For this review, take the finished solid that the model builds, in its own axes (mm). Face numbers are marked on the shaded views. A direction names the side the tool comes from. Coordinates: 2 decimals unless noted, no trailing zeros. Write each loop counter-clockwise with the first axis right and the second up, starting at its lowest first coordinate (ties: lowest second). Pieces come first, ordered by that corner, then holes. Notation, with made-up numbers: M 54.5,74 L 80.5,74 A13 ccw 80.5,92 Z; hole C 80.5,-17 d10. An arc over 180 degrees is marked long. Return JSON: item names as keys, results as strings.
```python
from build123d import *

# Parameters (mm, degrees)
SKETCH1_W           = 40
SKETCH1_H           = 40
BOSS_EXTRUDE1_DEPTH = 40
CUT_EXTRUDE1_DEPTH  = 40
CUT_EXTRUDE2_DEPTH  = 40
CUT_EXTRUDE10_DEPTH = 40
CUT_EXTRUDE11_DEPTH = 40
CUT_EXTRUDE12_DEPTH = 40


with BuildPart() as part:
    # Sketch1 → Boss-Extrude1 (new body)
    with BuildSketch(Plane.XY):
        with Locations((20, 20)):
            Rectangle(SKETCH1_W, SKETCH1_H)
    extrude(amount=BOSS_EXTRUDE1_DEPTH)

    # Sketch2 → Cut-Extrude1 (cut)
    with BuildSketch(Plane.XY.offset(40)):
        Polygon((0, 0), (20, 40), (0, 40), align=None)
    extrude(amount=-CUT_EXTRUDE1_DEPTH, mode=Mode.SUBTRACT)

    # Sketch3 → Cut-Extrude2 (cut)
    with BuildSketch(Plane(origin=(0, 0, 0), x_dir=(-1, 0, 0), z_dir=(0, -1, 0))):
        Polygon((0, 0), (-20, -20), (-20, -40), (0, -40), align=None)
    extrude(amount=-CUT_EXTRUDE2_DEPTH, mode=Mode.SUBTRACT)

    # Sketch12 → Cut-Extrude10 (cut)
    with BuildSketch(Plane.ZY.offset(-20)):
        Polygon((20, 40), (40, 0), (40, 40), align=None)
    extrude(amount=-CUT_EXTRUDE10_DEPTH, mode=Mode.SUBTRACT)

    # Sketch13 → Cut-Extrude11 (cut)
    with BuildSketch(Plane.XZ):
        Polygon((20, 40), (40, 20), (40, 40), align=None)
    extrude(amount=-CUT_EXTRUDE11_DEPTH, mode=Mode.SUBTRACT)

    # Sketch14 → Cut-Extrude12 (cut)
    with BuildSketch(Plane(origin=(26.666666667, 13.333333333, 26.666666667), x_dir=(-0.745355992, 0.298142397, 0.596284794), z_dir=(-0.666666667, -0.333333333, -0.666666667))):
        Polygon((-17.88854382, 35.77708764), (-17.88854382, -8.94427191), (8.94427191, -17.88854382), (8.94427191, 26.83281573), align=None)
    extrude(amount=-CUT_EXTRUDE12_DEPTH, mode=Mode.SUBTRACT)


solid = part.part
```
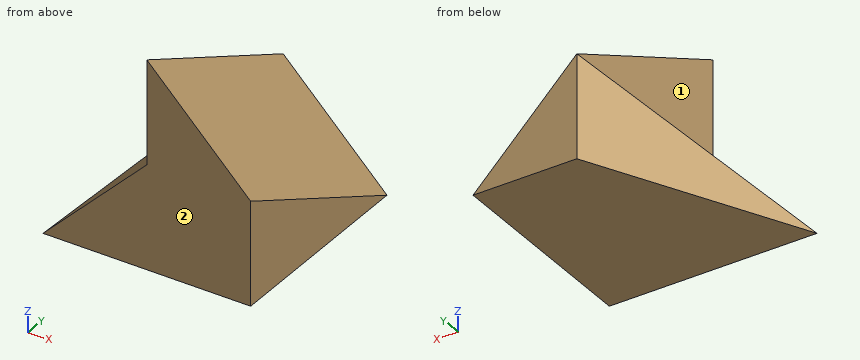
1. We need section B-B (y = 12.5). State the section outline as (x, z) points, plus the area to 3 significant figures.
Checks:
{"outline": "M 6.25,0 L 40,0 L 40,13.75 L 20,33.75 L 20,20 L 6.25,6.25 Z", "area": "655 mm2"}
2. Wall thickness on L1, parallel to Y at x = 29, z = 25.5; L2, parallel to X at y = 14, z = 12; L3, parallel to X at y = 33, z = 14: over which ranges is each line inside the solid? List them lowest first. Write a range as from..to.
Checks:
{"L1": "0..11", "L2": "12..40", "L3": "16.5..29.5"}
3. For the marked faces 1 and 2, list the 3-axis set-ups (+Z, -Z, +X, -X, +Y, -Y) from which the entire face can be reached by the end or side of a thin tool; tool diameter is ignored.
Checks:
{"face 1": "+Z, -X, +Y, -Y", "face 2": "+Z, -Z, +X, -X, -Y"}
4. Clearance check with flat-ended pins moving along their axes: pin 1 Ø8 at (y, z) = (18, 4) entering from -X; pin 2 Ø10 at (y, z) = (28.5, 30.5) entering from -X; pin 3 Ø3 at (x, z) = (15, 9.5) entering from +Y. State where each tip first meets the part, or that it passes through.
Checks:
{"pin 1": "x = 7", "pin 2": "x = 20", "pin 3": "y = 33"}
5. We need section A-A (z = 7.5). State the section outline as (x, y) points.
Checks:
{"outline": "M 7.5,0 L 40,0 L 40,25 L 32.5,40 L 20,40 L 7.5,15 Z"}
6. We need section D-D (z = 23.5). State the section outline as (x, y) points, plus the area to 3 significant figures.
Checks:
{"outline": "M 20,0 L 36.5,0 L 20,33 Z", "area": "272 mm2"}
7. We need section C-C (x = 21.5). State the section outline as (y, z) points, plus the area to 3 significant figures.
Checks:
{"outline": "M 0,0 L 40,0 L 40,18.5 L 0,38.5 Z", "area": "1,140 mm2"}
